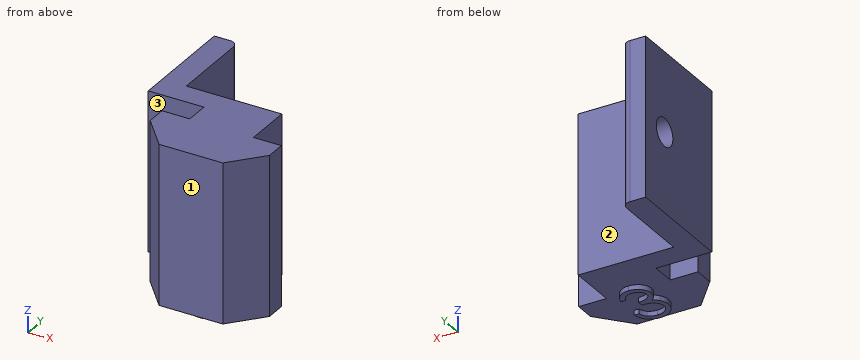
```python
from build123d import *

# Parameters (mm, degrees)
ESTRUSIONE_ESTRUSIONE1_DEPTH = 20
TAGLIO_ESTRUSIONE1_REACH     = 37.979
SCHIZZO6_R                   = 1.75
ESTRUSIONE_ESTRUSIONE4_DEPTH = 0.6


with BuildPart() as part:
    # Schizzo2 → Estrusione-Estrusione1 (new body)
    with BuildSketch(Plane.XY):
        with BuildLine():
            Line((-4, 9.5), (-11, 9.5))
            Line((-11, 9.5), (-11, 23.5))
            Line((-11, 23.5), (-9, 23.5))
            ThreePointArc((-9, 23.5), (-8.292893219, 23.207106781), (-8, 22.5))
            Line((-8, 22.5), (-8, 12.5))
            Line((-8, 12.5), (4, 12.5))
            Line((4, 12.5), (4, 9.5))
            Line((4, 9.5), (4, 6.5))
            Line((4, 6.5), (7.5, 6.5))
            Line((7.5, 6.5), (7.5, 4))
            Line((7.5, 4), (4, 0))
            Line((4, 0), (-4, 0))
            Line((-4, 0), (-7.5, 4))
            Line((-7.5, 4), (-7.5, 6.5))
            Line((-7.5, 6.5), (-4, 6.5))
            Line((-4, 6.5), (-4, 9.5))
        make_face()
    extrude(amount=-ESTRUSIONE_ESTRUSIONE1_DEPTH)

    # Schizzo6 → Taglio-Estrusione1 (cut, up to next)
    with BuildSketch(Plane.ZY.offset(11), mode=Mode.PRIVATE) as taglio_estrusione1_sk1:
        with Locations((-10, 19.5)):
            Circle(SCHIZZO6_R)
    taglio_estrusione1_tool1 = extrude(taglio_estrusione1_sk1.sketch, amount=-TAGLIO_ESTRUSIONE1_REACH, mode=Mode.PRIVATE) & part.part
    add(taglio_estrusione1_tool1.solids().sort_by_distance((-11, 19.5, -10))[0], mode=Mode.SUBTRACT)

    # Schizzo11 → Estrusione-Estrusione4 (add)
    with BuildSketch(Plane(origin=(0, 0, -20), x_dir=(-1, 0, 0), z_dir=(0, 0, -1))):
        with BuildLine():
            Line((-1.916666667, 6), (-2.5, 6))
            add(Edge.make_bspline(
                [(-2.5, 6), (-2.484196549, 6.065431756), (-2.453302094, 6.193345487), (-2.388863743, 6.376101829), (-2.318665127, 6.549045511), (-2.234371075, 6.708938219), (-2.142426246, 6.858993324), (-2.037084049, 6.995807413), (-1.923204564, 7.122860063), (-1.797243944, 7.235613218), (-1.665147858, 7.337714716), (-1.525054993, 7.424768393), (-1.379783905, 7.499656106), (-1.228328086, 7.561350822), (-1.070236625, 7.607826795), (-0.906938753, 7.641546577), (-0.738006538, 7.66344436), (-0.623332441, 7.665581492), (-0.565104167, 7.666666667)],
                knots=[0, 0, 0, 0, 1.162005537, 2.271625781, 3.343758855, 4.383309926, 5.390229558, 6.379919256, 7.361854164, 8.333198761, 9.295911338, 10.242430842, 11.177959212, 12.116337295, 13.062827104, 14.020064771, 14.994644689, 16, 16, 16, 16], degree=3))
            add(Edge.make_bspline(
                [(-0.565104167, 7.666666667), (-0.480264789, 7.664105239), (-0.312436625, 7.659038256), (-0.065876681, 7.612768588), (0.171887412, 7.539550485), (0.398253158, 7.438384992), (0.608515961, 7.313608553), (0.795597451, 7.165102613), (0.956961828, 6.995732482), (1.092337101, 6.80865772), (1.198333527, 6.608726059), (1.276493935, 6.402954339), (1.324077057, 6.191830678), (1.330243806, 6.049281445), (1.333333333, 5.977864583)],
                knots=[0, 0, 0, 0, 1.083050992, 2.142477498, 3.193116406, 4.255571735, 5.30263384, 6.308962982, 7.297363603, 8.282367274, 9.249857812, 10.179914175, 11.08814088, 12, 12, 12, 12], degree=3))
            add(Edge.make_bspline(
                [(1.333333333, 5.977864583), (1.331172379, 5.909137679), (1.326943725, 5.774649792), (1.291038272, 5.578309869), (1.230613784, 5.393261183), (1.146912796, 5.218724739), (1.038564203, 5.055807179), (0.907314909, 4.904141953), (0.752238537, 4.763056374), (0.634720509, 4.682234495), (0.57421875, 4.640625)],
                knots=[0, 0, 0, 0, 1.024540389, 2.004866551, 2.965041327, 3.920577974, 4.882998113, 5.874504559, 6.905732034, 8, 8, 8, 8], degree=3))
            add(Edge.make_bspline(
                [(0.57421875, 4.640625), (0.643363437, 4.607236967), (0.780359061, 4.541085617), (0.967095758, 4.411353496), (1.136611813, 4.261563137), (1.231147291, 4.144669639), (1.278645833, 4.0859375)],
                knots=[0, 0, 0, 0, 1.015518401, 2.012035669, 3.001164323, 4, 4, 4, 4], degree=3))
            add(Edge.make_bspline(
                [(1.278645833, 4.0859375), (1.309922612, 4.043115961), (1.37196399, 3.958174116), (1.448544267, 3.821606468), (1.518018337, 3.683525131), (1.572154458, 3.540229091), (1.614077354, 3.393379209), (1.644044271, 3.24272333), (1.662660533, 3.088138431), (1.665326558, 2.983558111), (1.666666667, 2.930989583)],
                knots=[0, 0, 0, 0, 1.025084078, 2.033381695, 3.024893161, 4.013698104, 4.991890475, 5.976764909, 6.982997093, 8, 8, 8, 8], degree=3))
            add(Edge.make_bspline(
                [(1.666666667, 2.930989583), (1.663333999, 2.83997153), (1.656684346, 2.658363755), (1.597248208, 2.390053558), (1.505109333, 2.127777625), (1.374260737, 1.876924352), (1.214792507, 1.64221793), (1.025071762, 1.43221907), (0.807254146, 1.251707377), (0.56432937, 1.100888382), (0.301140417, 0.980326526), (0.019642889, 0.896648418), (-0.276107211, 0.842148704), (-0.478920764, 0.836304519), (-0.58203125, 0.833333333)],
                knots=[0, 0, 0, 0, 0.955779014, 1.907060117, 2.875433937, 3.871313158, 4.872415639, 5.851225146, 6.836215519, 7.83643374, 8.849228613, 9.86973379, 10.916971861, 12, 12, 12, 12], degree=3))
            add(Edge.make_bspline(
                [(-0.58203125, 0.833333333), (-0.651524236, 0.834945729), (-0.78826326, 0.838118387), (-0.9892869, 0.859807218), (-1.181170056, 0.899420085), (-1.364172166, 0.952726223), (-1.538455805, 1.020310887), (-1.703489143, 1.104474184), (-1.860287517, 1.203481259), (-2.007371283, 1.318500779), (-2.144722909, 1.447166124), (-2.268692254, 1.591761428), (-2.381346155, 1.74961375), (-2.479668199, 1.922556569), (-2.568136825, 2.108354904), (-2.640901459, 2.309387829), (-2.704946086, 2.523858156), (-2.73472252, 2.673316816), (-2.75, 2.75)],
                knots=[0, 0, 0, 0, 1.048658725, 2.063410685, 3.046034179, 4.001477787, 4.936774919, 5.862367409, 6.792675028, 7.730719943, 8.675894397, 9.627829632, 10.600096036, 11.597688215, 12.626045268, 13.701542398, 14.82072376, 16, 16, 16, 16], degree=3))
            Line((-2.75, 2.75), (-2.166666667, 2.75))
            add(Edge.make_bspline(
                [(-2.166666667, 2.75), (-2.151469125, 2.699951833), (-2.121908588, 2.602603799), (-2.071590606, 2.462500375), (-2.014263815, 2.33406399), (-1.952765349, 2.216352478), (-1.888176806, 2.108206588), (-1.815906231, 2.012485974), (-1.74130639, 1.924986312), (-1.685073305, 1.875689176), (-1.657552083, 1.8515625)],
                knots=[0, 0, 0, 0, 1.198163088, 2.33053128, 3.407730985, 4.417276592, 5.372219308, 6.28897303, 7.162600585, 8, 8, 8, 8], degree=3))
            add(Edge.make_bspline(
                [(-1.657552083, 1.8515625), (-1.621158441, 1.823504166), (-1.548483496, 1.767474107), (-1.430056781, 1.695971082), (-1.305507707, 1.634014892), (-1.172137598, 1.586688029), (-1.032824452, 1.54661523), (-0.885316488, 1.520391409), (-0.730915085, 1.502399091), (-0.625489239, 1.500811361), (-0.571614583, 1.5)],
                knots=[0, 0, 0, 0, 0.946170439, 1.889420265, 2.845303464, 3.807233317, 4.801018734, 5.828864929, 6.890507805, 8, 8, 8, 8], degree=3))
            add(Edge.make_bspline(
                [(-0.571614583, 1.5), (-0.51078665, 1.501143824), (-0.391842877, 1.503380473), (-0.218283853, 1.523949643), (-0.053170021, 1.553906125), (0.101665412, 1.600173093), (0.24825064, 1.657337532), (0.384530847, 1.729113142), (0.512295044, 1.813324768), (0.629906797, 1.909040348), (0.735662739, 2.013823125), (0.828778978, 2.123418828), (0.907939064, 2.237365369), (0.97179428, 2.356293307), (1.022216731, 2.479710161), (1.056542675, 2.607962273), (1.080409774, 2.740000053), (1.082353483, 2.829753852), (1.083333333, 2.875)],
                knots=[0, 0, 0, 0, 1.217147791, 2.380027433, 3.494444702, 4.572153297, 5.609568379, 6.639424714, 7.649109417, 8.668170816, 9.669597737, 10.625200337, 11.543417969, 12.441394052, 13.322311151, 14.205496177, 15.095365482, 16, 16, 16, 16], degree=3))
            add(Edge.make_bspline(
                [(1.083333333, 2.875), (1.080491345, 2.935563915), (1.074821509, 3.056390388), (1.031534147, 3.234151597), (0.960333399, 3.405423649), (0.860655878, 3.567284402), (0.739318097, 3.71729679), (0.597497555, 3.851143829), (0.43401656, 3.961588284), (0.283551089, 4.037895789), (0.150272941, 4.089964642), (0.036215798, 4.124646719), (-0.091475036, 4.154014937), (-0.231255399, 4.181337727), (-0.384178515, 4.204591659), (-0.5500779, 4.223983603), (-0.728987171, 4.239500107), (-0.852842194, 4.246429284), (-0.916666667, 4.25)],
                knots=[0, 0, 0, 0, 1.07054697, 2.135767047, 3.216561865, 4.33974944, 5.486079747, 6.621378074, 7.775625952, 8.963672916, 9.598146892, 10.304877434, 11.070270905, 11.915000392, 12.823868403, 13.805723172, 14.86925407, 16, 16, 16, 16], degree=3))
            Line((-0.916666667, 4.25), (-0.916666667, 4.916666667))
            add(Edge.make_bspline(
                [(-0.916666667, 4.916666667), (-0.836250216, 4.918031302), (-0.678734144, 4.920704288), (-0.448644721, 4.95303345), (-0.228622855, 4.997754616), (-0.02354462, 5.066255688), (0.163374419, 5.145816239), (0.325539394, 5.238398914), (0.460678382, 5.34131202), (0.568134658, 5.456144008), (0.648974654, 5.579300525), (0.708081563, 5.707660032), (0.742996455, 5.842347574), (0.747657265, 5.934266243), (0.75, 5.98046875)],
                knots=[0, 0, 0, 0, 1.321986639, 2.589447074, 3.816329219, 5.01088745, 6.139805852, 7.153945165, 8.075214402, 8.924034688, 9.728124013, 10.488707548, 11.240355623, 12, 12, 12, 12], degree=3))
            add(Edge.make_bspline(
                [(0.75, 5.98046875), (0.74923038, 6.014413134), (0.747699256, 6.081943876), (0.728390026, 6.180604717), (0.69937395, 6.276249331), (0.659483024, 6.368470979), (0.606089798, 6.456630059), (0.542192966, 6.541478178), (0.466109351, 6.622530911), (0.37892495, 6.698080076), (0.285303026, 6.770080088), (0.182696301, 6.831205413), (0.074198534, 6.883474814), (-0.040310397, 6.926578176), (-0.161202096, 6.959002568), (-0.28790856, 6.982283416), (-0.420671401, 6.996839061), (-0.511247475, 6.99893469), (-0.557291667, 7)],
                knots=[0, 0, 0, 0, 0.884392785, 1.759457502, 2.611959086, 3.489218968, 4.37281399, 5.2945488, 6.255912374, 7.266815255, 8.301784654, 9.332968512, 10.37626691, 11.440494194, 12.520033166, 13.637162961, 14.798855837, 16, 16, 16, 16], degree=3))
            add(Edge.make_bspline(
                [(-0.557291667, 7), (-0.631301907, 6.997416042), (-0.775861121, 6.992368971), (-0.984260252, 6.948163375), (-1.177996158, 6.877632648), (-1.326082253, 6.793442755), (-1.435435605, 6.710334806), (-1.51357849, 6.637753232), (-1.590316581, 6.557092273), (-1.660601409, 6.463383862), (-1.731681652, 6.362974109), (-1.79639298, 6.2507587), (-1.859275266, 6.129664825), (-1.897165715, 6.044058647), (-1.916666667, 6)],
                knots=[0, 0, 0, 0, 1.472543308, 2.876219568, 4.221790263, 5.565193594, 6.249813518, 6.953379497, 7.687249741, 8.463570142, 9.283606569, 10.136032583, 11.040678096, 12, 12, 12, 12], degree=3))
        make_face()
    extrude(amount=ESTRUSIONE_ESTRUSIONE4_DEPTH)


solid = part.part
```
Model file for the job. Use its own axes, mm. Face numbers are marked on the shaded views. A direction names the side the tool comes from. Round coordinates to 2 decimals unless told otherwise and drop trailing zeros. Write each loop counter-clockwise with the first axis right and the second up, starting at its lowest first coordinate (ties: lowest second). Pieces come first, ordered by that corner, then holes. Notation, with made-up numbers: (-27.5, 5) -> (-12.5, 5) arc R28 ccw to (-12.5, 25) -> close; hole circle Ø8 at (-30, 11.25). An arc over 180 degrees is marked (long way). Answer as CSV lines item,"result".
1. Pin check, flat tips, straight feed: pin 1 Ø1 at (y, z) = (8.5, -2.5) entering from -X; pin 2 Ø2 at (y, z) = (5.5, -10.5) entering from -X; pin 3 Ø8 at (y, z) = (18, -8) entering from +X; pin 4 Ø3 at (y, z) = (19.5, -10) entering from -X. Stop position of each tip, or through.
Resolved:
pin 1,"x = -4"
pin 2,"x = -7.5"
pin 3,"x = -8"
pin 4,"through"
2. Drill centre lines: line 1 (Y direction, x = -9.3, z = -10); line 2 (Z direction, x = -0.25, y = 12); line 3 (X direction, y = 17.25, z = -4.5). Where is each one in solid material? Low to high.
Resolved:
line 1,"9.5 to 17.75, 21.25 to 23.5"
line 2,"-20 to 0"
line 3,"-11 to -8"
3. Slice it at D-D, the plane z = -14.25. List the corners of the cut face in (x, y), plus the area to 3 significant figures.
Resolved:
outline,"(-11, 9.5) -> (-4, 9.5) -> (-4, 6.5) -> (-7.5, 6.5) -> (-7.5, 4) -> (-4, 0) -> (4, 0) -> (7.5, 4) -> (7.5, 6.5) -> (4, 6.5) -> (4, 12.5) -> (-8, 12.5) -> (-8, 22.5) arc R1 ccw to (-9, 23.5) -> (-11, 23.5) -> close"
area,"185 mm²"
4. Slice it at C-C, the plane x = -6. List the corners of the cut face in (y, z), plus the area to 3 significant figures.
Resolved:
outline,"(2.29, -20) -> (6.5, -20) -> (6.5, 0) -> (2.29, 0) -> close; (9.5, -20) -> (12.5, -20) -> (12.5, 0) -> (9.5, 0) -> close"
area,"144 mm²"
5. Slice it at A-A, the plane z = -10. List the corners of the cut face in (x, y), plus the area to 3 significant figures.
Resolved:
outline,"(-11, 9.5) -> (-4, 9.5) -> (-4, 6.5) -> (-7.5, 6.5) -> (-7.5, 4) -> (-4, 0) -> (4, 0) -> (7.5, 4) -> (7.5, 6.5) -> (4, 6.5) -> (4, 12.5) -> (-8, 12.5) -> (-8, 17.75) -> (-11, 17.75) -> close; (-11, 21.25) -> (-8, 21.25) -> (-8, 22.5) arc R1 ccw to (-9, 23.5) -> (-11, 23.5) -> close"
area,"175 mm²"
6. Slice it at B-B, the plane y = 19.5. List the corners of the cut face in (x, z).
Resolved:
outline,"(-11, -20) -> (-8, -20) -> (-8, -11.75) -> (-11, -11.75) -> close; (-11, -8.25) -> (-8, -8.25) -> (-8, 0) -> (-11, 0) -> close"
7. Tool access for the marked faces 1, 2 and 3: list every direction of +Z, -Z, +X, -X, +Y, -Y with a clear straight run to the whole face (end or side of a thin tool).
Resolved:
face 1,"+Z, -Z, +X, -X, -Y"
face 2,"+Z, -Z, +X, +Y"
face 3,"+Z, -Z, -X"
